```python
from build123d import *

# Parameters (mm, degrees)
PAD_DEPTH       = 10
SKETCH_W        = 60
SKETCH_H        = 93
POCKET_DEPTH    = 8
SKETCH005_W     = 12
SKETCH005_H     = 8
POCKET003_DEPTH = 2


with BuildPart() as part:
    # Sketch001 → Pad (new body)
    with BuildSketch(Plane.XY):
        with BuildLine():
            ThreePointArc((0, 2), (-1.414214, 1.414214), (-2, 0))
            Line((-2, 0), (-2, -93))
            ThreePointArc((-2, -93), (-1.414207, -94.414201), (0, -94.999981))
            Line((0, -94.999981), (60, -94.999981))
            ThreePointArc((60, -94.999981), (61.414214, -94.414194), (62, -92.99998))
            Line((62, 0), (62, -92.99998))
            ThreePointArc((62, 0), (61.414214, 1.414214), (60, 2))
            Line((0, 2), (60, 2))
        make_face()
    extrude(amount=PAD_DEPTH)

    # Sketch (on Face10 of Pad) → Pocket (cut)
    with BuildSketch(Plane.XY.offset(10)):
        with Locations((30, -46.5)):
            Rectangle(SKETCH_W, SKETCH_H)
    extrude(amount=-POCKET_DEPTH, mode=Mode.SUBTRACT)

    # Sketch005 (on Face2 of Pocket) → Pocket003 (cut)
    with BuildSketch(Plane.YZ.offset(62)):
        with Locations((-13, 6)):
            Rectangle(SKETCH005_W, SKETCH005_H)
    extrude(amount=-POCKET003_DEPTH, mode=Mode.SUBTRACT)


solid = part.part
```
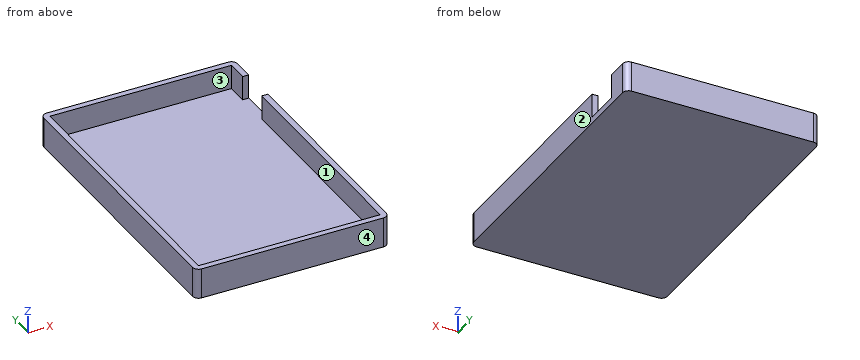
Source: CAD feature listing. Evaluate the final solid. Frame: model axes, mm. Face numbers are marked on the shaded views. Give positions to 0.01 mm unless a question says otherwise; leave off trailing zeros. Loops run counter-clockwise (first coordinate to the right, second up) from the corner with the lowest first, then second, coordinate; pieces in that order, holes last. Notation, with made-up numbers: (-8, 62) -> (17, 62) arc R19 cw to (17, 78) -> close; hole circle Ø9 at (50.5, 48). An arc over 180 degrees is marked (long way). Put each result on its own line as item: value. Start each with the question number.
1) Cut plane C-C (z = 4.5). Return loops of the section in (x, y).
2) Cut plane B-B (y = -13). Return loops of the section in (x, z).
3) Material intervals for probe 1 along Y at (x, z) = (39, 8.25); probe 2 along X at (y, z) = (-71, 9); probe 3 along Z at (x, y) = (45, -79.5), sorted ascending.
4) Draft query along Y for the marked faces 1, 2, 3 and 4. Return one class per face: released by +Y, released by -Y, zero draft, split by the parting line, or undercut.
5) Cut plane D-D (y = -35). Return loops of the section in (x, z).
6) Cut plane A-A (x = 33). Return loops of the section in (y, z), then the cut area to 3 significant figures.
7) Contact query for flat-ended pins moving along their axis: P1, Ø1, axis at x = 61, z = 7.5, coming from the -Y side; P2, Ø0.6, axis at x = 60.5, z = 4, coming from the +Y side; P3, Ø1.5, axis at x = 19.5, y = -59.5, coming from the +Z side. Output: stop coordinate, or through.
Results are:
1. outline: (-2, -93) arc R2 ccw to (0, -95) -> (60, -95) arc R2 ccw to (62, -93) -> (62, -19) -> (60, -19) -> (60, -93) -> (0, -93) -> (0, 0) -> (60, 0) -> (60, -7) -> (62, -7) -> (62, 0) arc R2 ccw to (60, 2) -> (0, 2) arc R2 ccw to (-2, 0) -> close
2. outline: (-2, 0) -> (62, 0) -> (62, 2) -> (0, 2) -> (0, 10) -> (-2, 10) -> close
3. probe 1: y = -95 to -93, 0 to 2
3. probe 2: x = -2 to 0, 60 to 62
3. probe 3: z = 0 to 2
4. face 1: undercut
4. face 2: zero draft
4. face 3: undercut
4. face 4: released by -Y
5. outline: (-2, 0) -> (62, 0) -> (62, 10) -> (60, 10) -> (60, 2) -> (0, 2) -> (0, 10) -> (-2, 10) -> close
6. outline: (-95, 0) -> (2, 0) -> (2, 10) -> (0, 10) -> (0, 2) -> (-93, 2) -> (-93, 10) -> (-95, 10) -> close
6. area: 226 mm2
7. P1: stops at y = -94.94
7. P2: stops at y = 1.99
7. P3: stops at z = 2
